Geometry check sheet. Reference: the model listing, model coordinates, mm. Face numbers are marked on the shaded views. A direction names the side the tool comes from. Coordinates: 2 decimals unless noted, no trailing zeros. Loops run counter-clockwise (first coordinate to the right, second up) from the corner with the lowest first, then second, coordinate; pieces in that order, holes last. Notation, with made-up numbers: M -14,82.5 L 45,82.5 A27 ccw 45,101.5 Z; hole C 37.25,78 d8. An arc over 180 degrees is marked long. Use CSV: the item, a comma, the result in double quotes.
```python
from build123d import *

# Parameters (mm, degrees)
SKETCH2_W          = 162.317604445
SKETCH2_H          = 55.549243825
CUT_EXTRUDE1_DEPTH = 15.875
SKETCH3_W          = 6.35
SKETCH3_H          = 3.175
CHAMFER1_SIZE      = 1.27


with BuildPart() as part:
    # Sketch1 → Revolve1 (revolve)
    with BuildSketch(Plane.XY, mode=Mode.PRIVATE) as revolve1_sk:
        Polygon((0, 31.75), (0, 6.477), (44.45, 6.477), (44.45, 12.7), (106.045, 12.7), (106.045, 19.05), (6.35, 19.05), (6.35, 31.75), align=None)
    revolve(revolve1_sk.sketch.rotate(Axis((0, 0, 0), (1, 0, 0)), 90), axis=Axis((0, 0, 0), (1, 0, 0)))

    # Sketch2 → Cut-Extrude1 (cut)
    with BuildSketch(Plane(origin=(106.045, 0, 0), x_dir=(0, 0, -1), z_dir=(1, 0, 0))):
        with Locations((1.710934167, 44.284621913)):
            Rectangle(SKETCH2_W, SKETCH2_H)
    extrude(amount=-CUT_EXTRUDE1_DEPTH, mode=Mode.SUBTRACT)

    # Sketch3 → Cut-Revolve1 (revolve, cut)
    with BuildSketch(Plane.XY, mode=Mode.PRIVATE) as cut_revolve1_sk:
        with Locations((96.266, 18.0975)):
            Rectangle(SKETCH3_W, SKETCH3_H)
    revolve(cut_revolve1_sk.sketch.rotate(Axis((0, 0, 0), (1, 0, 0)), 90), axis=Axis((0, 0, 0), (1, 0, 0)), mode=Mode.SUBTRACT)

    # Chamfer1
    chamfer1_edges = [part.edges().sort_by_distance(p)[0] for p in [
        (106.045, -19.05, 0),
    ]]
    chamfer(chamfer1_edges, length=CHAMFER1_SIZE)


solid = part.part
```
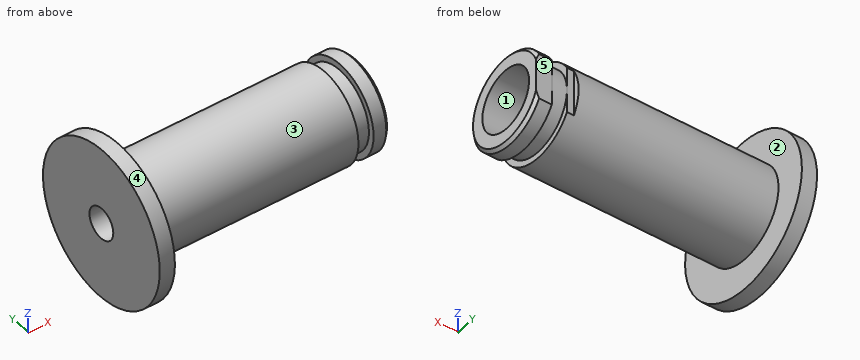
1. Thickness scan on line 1 (Y direction, x = 28, z = 0); line 2 (Y direction, x = 73, z = 0); line 3 (X direction, y = 6.5, z = 16.5) (3 decimals). Record the ranges inside material, lowest first. Write a range as [from, to].
The answers:
line 1,"[-19.05, -6.48], [6.48, 19.05]"
line 2,"[-19.05, -12.7], [12.7, 19.05]"
line 3,"[0, 93.091], [99.441, 106.045]"
2. Section check A-A, the plane y = 0. Record the cut outline in (x, z) (3 decimals).
The answers:
outline,"M 0,-31.75 L 6.35,-31.75 L 6.35,-19.05 L 93.091,-19.05 L 93.091,-16.51 L 99.441,-16.51 L 99.441,-19.05 L 104.775,-19.05 L 106.045,-17.78 L 106.045,-12.7 L 44.45,-12.7 L 44.45,-6.477 L 0,-6.477 Z; M 0,6.477 L 44.45,6.477 L 44.45,12.7 L 106.045,12.7 L 106.045,17.78 L 104.775,19.05 L 99.441,19.05 L 99.441,16.51 L 93.091,16.51 L 93.091,19.05 L 6.35,19.05 L 6.35,31.75 L 0,31.75 Z"
3. Gauge pin test, flat ends, axial feed: P1, Ø10, axis at x = 56.5, z = 15, coming from the +Y side; P2, Ø20.5, axis at y = 0, z = 0, coming from the -X side; P3, Ø2, axis at x = 94.5, z = -11.5, coming from the -Y side; P4, Ø2, axis at y = 18, z = -3, coming from the +X side. Record the tip position at first contact, or that the pin passes through.
The answers:
P1,"y = 16.21"
P2,"x = 0"
P3,"y = -12.74"
P4,"x = 90.17"
4. Section check C-C, the plane z = 20.5. Record the cut outline in (x, y), plus the area to 3 significant figures.
The answers:
outline,"M 0,-24.24 L 6.35,-24.24 L 6.35,24.24 L 0,24.24 Z"
area,"308 mm^2"
5. Section check B-B, the plane x = 61. Record the cut outline in (y, z), plus the area to 3 significant figures.
The answers:
outline,"C 0,0 d38.1; hole C 0,0 d25.4"
area,"633 mm^2"
6. Section check D-D, the plane x = 29.5. Record the cut outline in (y, z).
The answers:
outline,"C 0,0 d38.1; hole C 0,0 d12.95"
7. Release check for a two-part mould opening along Z. For the marked faces 1, 2 and 3 record: +Z half, -Z half, draft (parallel to the pull), parting line (faces both ways), or undercut.
The answers:
face 1,"undercut"
face 2,"draft"
face 3,"parting line"
8. Set-up check for the marked faces 4 and 5: record each of +Z, -Z, +X, -X, +Y, -Y from which the full face is reachable in a straight line by a thin tool's end or side.
The answers:
face 4,"+X, -X"
face 5,"+Z, -Z, +X, +Y"
